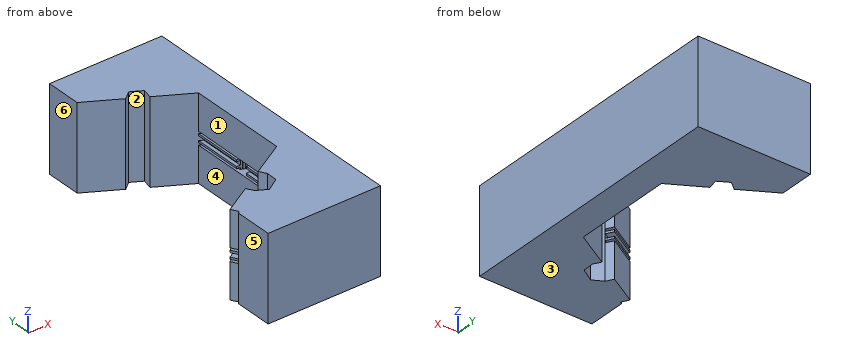
```python
from build123d import *

# Parameters (mm, degrees)
BOSS_EXTRUDE1_DEPTH      = 10
BOSS_EXTRUDE1_DEPTH_BACK = 11
SKETCH2_W                = 0.5
SKETCH2_H                = 33.789751219
SKETCH2_W_2              = 8.9
SKETCH2_H_2              = 33.710181146
BOSS_EXTRUDE2_DEPTH      = 0.9
SKETCH4_W                = 3.2
SKETCH4_H                = 3.035313039
CUT_EXTRUDE1_DEPTH       = 0.9
SKETCH5_W                = 8.9
SKETCH5_H                = 5.924846374
SKETCH5_H_2              = 8.259633143
BOSS_EXTRUDE3_DEPTH      = 3.9
SKETCH6_W                = 10.051459914
SKETCH6_H                = 8.9
SKETCH6_W_2              = 8.141320355
SKETCH6_W_3              = 10.023699464
SKETCH6_H_2              = 0.55
SKETCH6_H_3              = 0.5
SKETCH6_W_4              = 8.105756988
BOSS_EXTRUDE4_DEPTH      = 2


with BuildPart() as part:
    # Sketch1 → Boss-Extrude1 (new body, two sides)
    with BuildSketch(Plane.XY) as boss_extrude1_sk:
        Polygon((0.795322437, -25.455965093), (8.355079741, -21.091337178), (10.890469069, -22.462482859), (14.044123283, -20.446434454), (14.129516604, -17.757464501), (22.479597834, -12.936542855), (22.479597834, -1.543644942), (23.016460709, -1.543644942), (23.016460709, -1.327475501), (23.549450475, -1.327475501), (24.148188576, -0.947681864), (24.148188576, 0.979689608), (23.549450475, 1.278840764), (23.016460709, 1.278840764), (23.016460709, 1.491668097), (22.479597834, 1.491668097), (22.479597834, 13.01230949), (13.267337289, 18.286375916), (13.8113599, 20.713241045), (11.090051556, 22.271204034), (9.1144107, 20.663947694), (0.795322437, 25.426668406), (0.795322437, 34.137830746), (28.694115234, 34.137830746), (28.694115234, -34.851518664), (0.795322437, -34.851518664), align=None)
    extrude(amount=BOSS_EXTRUDE1_DEPTH)
    extrude(boss_extrude1_sk.sketch, amount=-BOSS_EXTRUDE1_DEPTH_BACK)

    # Sketch2 → Boss-Extrude2 (add)
    with BuildSketch(Plane.ZY.offset(-22.479597834)):
        with Locations((-1.3, 1.391500307)):
            Rectangle(SKETCH2_W, SKETCH2_H)
        with Locations((-6.55, 1.391500307)):
            Rectangle(SKETCH2_W_2, SKETCH2_H)
        with Locations((5.55, 1.431285343)):
            Rectangle(SKETCH2_W_2, SKETCH2_H_2)
        with Locations((0.3, 1.431285343)):
            Rectangle(SKETCH2_W, SKETCH2_H_2)
    extrude(amount=BOSS_EXTRUDE2_DEPTH)

    # Sketch4 → Cut-Extrude1 (cut)
    with BuildSketch(Plane.ZY.offset(-21.579597834)):
        with Locations((-0.5, -0.025988422)):
            Rectangle(SKETCH4_W, SKETCH4_H)
    extrude(amount=-CUT_EXTRUDE1_DEPTH, mode=Mode.SUBTRACT)

    # Sketch5 → Boss-Extrude3 (add)
    with BuildSketch(Plane.ZY.offset(-21.579597834)):
        with Locations((5.55, -0.357470261)):
            Rectangle(SKETCH5_W, SKETCH5_H)
        with Locations((-6.55, -0.62015136)):
            Rectangle(SKETCH5_W, SKETCH5_H_2)
    extrude(amount=-BOSS_EXTRUDE3_DEPTH)

    # Sketch6 → Boss-Extrude4 (add)
    with BuildSketch(Plane(origin=(11.221586833, -19.436358537, 0), x_dir=(0.866025404, 0.5, 0), z_dir=(-0.5, 0.866025404, 0))):
        with Locations((8.383518028, -5.55)):
            Rectangle(SKETCH6_W, SKETCH6_H)
        with Locations((8.383518028, 6.55)):
            Rectangle(SKETCH6_W, SKETCH6_H)
        with Locations((-7.38061746, -5.55)):
            Rectangle(SKETCH6_W_2, SKETCH6_H)
        with Locations((8.397398253, -0.275)):
            Rectangle(SKETCH6_W_3, SKETCH6_H_2)
        with Locations((8.397398253, 1.3)):
            Rectangle(SKETCH6_W_3, SKETCH6_H_3)
        with Locations((-7.398399144, -0.275)):
            Rectangle(SKETCH6_W_4, SKETCH6_H_2)
        with Locations((-7.398399144, 1.3)):
            Rectangle(SKETCH6_W_4, SKETCH6_H_3)
        with Locations((-7.38061746, 6.55)):
            Rectangle(SKETCH6_W_2, SKETCH6_H)
    extrude(amount=BOSS_EXTRUDE4_DEPTH)


solid = part.part
```
The listing builds one solid part. Answer for the finished solid, in the listing's coordinates (mm). Face numbers are marked on the shaded views. A direction names the side the tool comes from. Round coordinates to 2 decimals unless told otherwise and drop trailing zeros. Loops run counter-clockwise (first coordinate to the right, second up) from the corner with the lowest first, then second, coordinate; pieces in that order, holes last.
1) Given P1, Ø12, axis at y = 22, z = -9, coming from the -X side; P2, Ø0.6, axis at y = -4.5, z = -2, coming from the -X side; P3, Ø1, axis at y = 20.5, z = 6.5, coming from the -X side, each flat-ended and moving along its own axis, determine where each tip first touches the part or whether it passes through.
Outcome:
P1: stops at x = 0.8
P2: stops at x = 21.58
P3: stops at x = 8.53
2) A cutting plane is placed at A-A on x = 6. Determine the outline of the cut face in (y, z), plus the area to 3 significant figures.
Outcome:
outline: (-34.85, -11) - (-20.14, -11) - (-20.14, -2.1) - (-22.45, -2.1) - (-22.45, -1.55) - (-20.14, -1.55) - (-20.14, -1.05) - (-22.45, -1.05) - (-22.45, 0) - (-20.14, 0) - (-20.14, 0.55) - (-22.45, 0.55) - (-22.45, 1.1) - (-20.14, 1.1) - (-20.14, 10) - (-34.85, 10) - close; (22.45, -11) - (34.14, -11) - (34.14, 10) - (22.45, 10) - close
area: 549 mm2
3) For a pull along X with two mould halves and no side action, classify the marked faces 1, 2 and 3 as released by +X, released by -X, zero draft, split by the parting line, or undercut.
Outcome:
face 1: released by -X
face 2: undercut
face 3: zero draft
4) A cutting plane is placed at D-D on x = 18.25. Determine the outline of the cut face in (y, z).
Outcome:
outline: (-34.85, -11) - (-13.07, -11) - (-13.07, -2.1) - (-15.38, -2.1) - (-15.38, -1.55) - (-13.07, -1.55) - (-13.07, -1.05) - (-15.38, -1.05) - (-15.38, 0) - (-13.07, 0) - (-13.07, 0.55) - (-15.38, 0.55) - (-15.38, 1.1) - (-13.07, 1.1) - (-13.07, 10) - (-34.85, 10) - close; (15.43, -11) - (34.14, -11) - (34.14, 10) - (15.43, 10) - close
5) For the marked faces 4, 5 and 6, determine the directions among +Z, -Z, +X, -X, +Y, -Y from which every point of the face is accessible in a straight line to the end or side of a thin tool.
Outcome:
face 4: +Z, -Z, -X
face 5: +Z, -Z, -X, -Y
face 6: +Z, -Z, -X, +Y
6) Consider line 1 (Y direction, x = 22.5, z = -1.5); line 2 (Y direction, x = 20.75, z = -9); line 3 (X direction, y = -18, z = -8.25). Determine where each line is inside the solid, lowest interval first.
Outcome:
line 1: y = -34.85 to -1.54, 1.49 to 34.14
line 2: y = -34.85 to -11.63, 14 to 34.14
line 3: x = 14.12 to 28.69
7) A cutting plane is placed at B-B on z = -6.75. Determine the outline of the cut face in (x, y).
Outcome:
outline: (0.3, -23.43) - (1.3, -25.16) - (0.8, -25.46) - (0.8, -34.85) - (28.69, -34.85) - (28.69, 34.14) - (0.8, 34.14) - (0.8, 25.43) - (9.11, 20.66) - (11.09, 22.27) - (13.81, 20.71) - (13.27, 18.29) - (21.58, 13.53) - (21.58, -11.15) - (13.13, -16.03) - (14.13, -17.76) - (14.04, -20.45) - (10.89, -22.46) - (8.36, -21.09) - (7.36, -19.36) - close
8) A cutting plane is placed at C-C on y = -3. Determine the outline of the cut face in (x, z), plus the area to 3 significant figures.
Outcome:
outline: (21.58, -11) - (28.69, -11) - (28.69, 10) - (21.58, 10) - (21.58, 1.1) - (22.48, 1.1) - (22.48, 0.55) - (21.58, 0.55) - (21.58, 0.05) - (22.48, 0.05) - (22.48, -1.05) - (21.58, -1.05) - (21.58, -1.55) - (22.48, -1.55) - (22.48, -2.1) - (21.58, -2.1) - close
area: 147 mm2
